from build123d import *

# Parameters (mm, degrees)
SKETCH_R         = 18
PAD_DEPTH        = 5.5
HOLE_D           = 5
HOLE_CSINK_D     = 10
HOLE_CSINK_ANGLE = 90
FILLET_R         = 0.9


with BuildPart() as part:
    # Sketch → Pad (new body)
    with BuildSketch(Plane.XY):
        with BuildLine():
            ThreePointArc((19, -40.129291), (0, 44.4), (-19, -40.129291))
            Line((-19, -40.129291), (-16, -40.129291))
            Line((-16, -40.129291), (-16, -36.129291))
            Line((-16, -36.129291), (16, -36.129291))
            Line((16, -36.129291), (16, -40.129291))
            Line((16, -40.129291), (19, -40.129291))
        make_face()
        Circle(SKETCH_R, mode=Mode.SUBTRACT)
    extrude(amount=PAD_DEPTH)

    # Hole (through all)
    with Locations(Plane.XY.offset(5.5)):
        with Locations((28, 25.911822), (-28, 25.911822), (-27, -19.077066), (27, -19.077066)):
            CounterSinkHole(HOLE_D / 2, HOLE_CSINK_D / 2, counter_sink_angle=HOLE_CSINK_ANGLE)

    # Fillet
    fillet_edges = [part.edges().sort_by_distance(p)[0] for p in [
        (0, 44.4, 5.5),
        (-18, 0, 5.5),
        (-17.5, -40.129291, 5.5),
        (-16, -38.129291, 5.5),
        (0, -36.129291, 5.5),
        (16, -38.129291, 5.5),
        (17.5, -40.129291, 5.5),
        (-16, -40.129291, 2.75),
        (16, -40.129291, 2.75),
        (-16, -36.129291, 2.75),
        (16, -36.129291, 2.75),
    ]]
    fillet(fillet_edges, radius=FILLET_R)


solid = part.part
Check sheet for the modelled part. Datum: model origin and axes. Units: mm. A direction names the side the tool comes from. Round coordinates to 2 decimals unless told otherwise and drop trailing zeros. Order: outer loops, then holes, each group sorted by start corner. A loop starts at its lowest first (then second) coordinate and runs counter-clockwise, first axis right, second up. Notation, with made-up numbers: M -5,33 L 17,33 A36 cw 17,67 Z; hole C 19.25,52.25 d11. An arc over 180 degrees is marked long. One line per item, written item: value. Start each with the question number.
1. Access from +Z, -Z, +X, -X, +Y, -Y to the whole of each face (thin tool, end or side, straight path). Record for faces 4 (the flat face through (16, -38, 2)), 5 (the cylindrical face through (28.54, 23.47, 1.48)).
2. Release check for a two-part mould opening along Y. For faces 1 (the cylindrical face through (-2.343, 17.847, 2.268)), 2 (the flat face through (-20, 3, 5.5)), 3 (the flat face through (-18, -40.129, 2)) record: released by +Y, released by -Y, zero draft, split by the parting line, or undercut.
3. Section check A-A on x = 0. Enter the section's corners in (y, z).
4. Section check C-C on x = -27. Give the number of separate pieces and of enclosed holes in the cut face, and give its area (3 significant figures).
5. Scan lines: line 1 along Y through (x, z) = (-27, 1.85); line 2 along X through (y, z) = (-21, 3.75); line 3 along Y through (x, z) = (-28, 2.2). Record each from-to range of solid material in increasing order.
6. Section check B-B on z = 1.9. Enter the section's corners in (x, y), and give its area (3 significant figures).
7. Gauge pin test, flat ends, axial feed: P1, Ø2, axis at y = 6, z = 2.5, coming from the -X side; P2, Ø1, axis at y = 0.5, z = 0.5, coming from the -X side; P3, Ø1.5, axis at y = -20, z = 1, coming from the -X side; P4, Ø2, axis at x = 9.5, y = 13.5, coming from the -Z side. Record the tip position at first contact, or that the pin passes through.
Results found:
1. face 4: +Z, -Z, -Y
1. face 5: +Z, -Z
2. face 1: undercut
2. face 2: zero draft
2. face 3: released by -Y
3. outline: M -36.13,0 L -18,0 L -18,4.6 A0.9 ccw -18.9,5.5 L -35.23,5.5 A0.9 ccw -36.13,4.6 Z; M 18,0 L 44.4,0 L 44.4,4.6 A0.9 ccw 43.5,5.5 L 18.9,5.5 A0.9 ccw 18,4.6 Z
4. separate pieces: 3
4. enclosed holes: 0
4. area: 322 mm^2
5. line 1: -35.25 to -21.58, -16.58 to 23.62, 28.2 to 35.25
5. line 2: -39.12 to -29.62, -24.38 to 24.38, 29.62 to 39.12
5. line 3: -34.46 to -21.37, -16.79 to 23.41, 28.41 to 34.46
6. outline: M -19,-40.13 L -16.9,-40.13 A0.9 ccw -16,-39.23 L -16,-37.03 A0.9 cw -15.1,-36.13 L 15.1,-36.13 A0.9 cw 16,-37.03 L 16,-39.23 A0.9 ccw 16.9,-40.13 L 19,-40.13 A44.4 ccw long Z; hole C -28,25.91 d5; hole C -27,-19.08 d5; hole C 0,0 d36; hole C 27,-19.08 d5; hole C 28,25.91 d5
6. area: 4,860 mm^2
7. P1: x = -44.12
7. P2: x = -44.4
7. P3: x = -40.01
7. P4: through
